Geometry: final body of the model. Coordinates: model frame, mm. A direction names the side the tool comes from. Give positions to 0.01 mm unless a question says otherwise; leave off trailing zeros. Write each loop counter-clockwise with the first axis right and the second up, starting at its lowest first coordinate (ties: lowest second). Pieces come first, ordered by that corner, then holes.
Autodesk Inventor part; units mm, degrees
ref_plane "YZ Plane" through (0, 0, 0) normal (1, 0, 0) x (0, 1, 0)
ref_plane "XZ Plane" through (0, 0, 0) normal (0, 1, 0) x (-1, 0, 0)
ref_plane "XY Plane" through (0, 0, 0) normal (0, 0, 1) x (1, 0, 0)
sketch "Sketch12" plane through (0, 0, 0) normal (0, 0, 1) x (1, 0, 0)
  line L0 (0, 0) -> (-12, 0)
  line L1 (-12, 0) -> (-12, 19)
  line L2 (-12, 19) -> (0, 19)
  line L3 (0, 19) -> (0, 0)
  dimension "d50" = 12
  dimension "d51" = 19
extrude "Extrusion8" add sketch "Sketch12" along normal blind 4
sketch "Sketch13" plane through (0, 0, 4) normal (0, 0, 1) x (1, 0, 0)
  line L0 (-12, 19) -> (-12, 0)
  line L1 (-12, 0) -> (-7, 0)
  line L2 (-7, 0) -> (-7, 2)
  line L3 (-7, 2) -> (-12, 2)
  line L4 (-12, 2) -> (-12, 0)
  line L5 (0, 19) -> (-12, 19)
  line L6 (0, 19) -> (-5, 19)
  line L7 (-5, 19) -> (-5, 17)
  line L8 (-5, 17) -> (0, 17)
  line L9 (0, 17) -> (0, 19)
  line L10 (-7, 2) -> (-5, 2)
  line L11 (-5, 2) -> (-5, 17)
  line L12 (-5, 17) -> (-7, 17)
  line L13 (-7, 17) -> (-7, 2)
  point P0 (0, 0)
  dimension "d54" = 5
  dimension "d55" = 2
  dimension "d56" = 5
  dimension "d57" = 2
extrude "Extrusion9" cut sketch "Sketch13" against normal blind 4 contours L13 L12 L11 L10
fillet "Fillet9" radius 1 4 edges at (-7, 17, 2) (-5, 17, 2) (-7, 2, 2) (-5, 2, 2)
properties part number "Rod"
Q1. Pull-direction query (X, two-part tool) for faces 3 (the flat face through (-12, 9, 2)), 4 (the flat face through (0, 10, 2)), 5 (the cylindrical face through (-6.699, 2.285, 1.972)); classes: released by +X, released by -X, zero draft, split by the parting line, or undercut.
Filled sheet:
face 3: released by -X
face 4: released by +X
face 5: undercut
Q2. Section C-C on y = 16.5. Output: boundary loops of the cut face in (x, z).
Filled sheet:
outline: (-12, 0) - (-6.87, 0) - (-6.87, 4) - (-12, 4) - close; (-5.13, 0) - (0, 0) - (0, 4) - (-5.13, 4) - close
Q3. Ray query, line 1 along X through (y, z) = (16, 2.1); line 2 along X through (y, z) = (16.75, 2.3). Return the intervals inside material, ascending.
Filled sheet:
line 1: x = -12 to -7, -5 to 0
line 2: x = -12 to -6.66, -5.34 to 0
Q4. Access query for faces 1 (the flat face through (-7, 10, 2)), 2 (the flat face through (-7.4, 9.6, 0)). Directions: +Z, -Z, +X, -X, +Y, -Y. A direction counts if a zero-diameter tool reaches every point of the face in a straight line with its end or side. Return the directions, or none.
Filled sheet:
face 1: +Z, -Z
face 2: -Z, +X, -X, +Y, -Y
Q5. Section B-B on y = 7. Output: boundary loops of the cut face in (x, z).
Filled sheet:
outline: (-12, 0) - (-7, 0) - (-7, 4) - (-12, 4) - close; (-5, 0) - (0, 0) - (0, 4) - (-5, 4) - close
Q6. Pin query (flat end, axial travel): P1, Ø1.5, axis at y = 2.5, z = 1, coming from the +X side. Return the tip coordinate at first contact, or that it passes through.
Filled sheet:
P1: stops at x = 0
